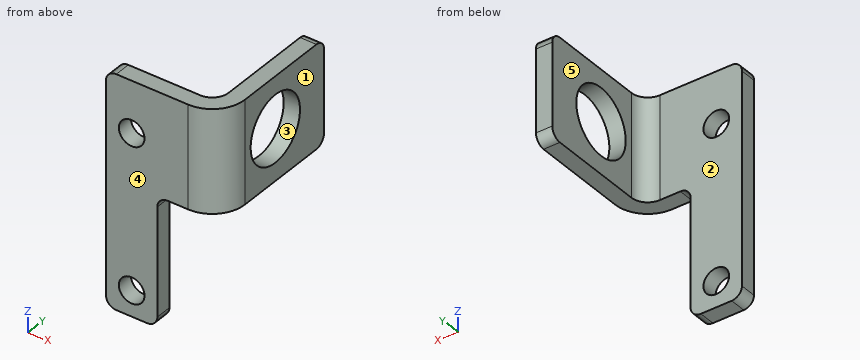
```python
from build123d import *

# Parameters (mm, degrees)
SKETCH2_W           = 10
SKETCH2_H           = 45
BOSS_EXTRUDE1_DEPTH = 3.175
CUT_EXTRUDE1_REACH  = 48.207
SKETCH4_R           = 2.5
EDGE_FLANGE2_DEPTH  = 20
CUT_EXTRUDE2_REACH  = 57.957
SKETCH15_R          = 6.5
FILLET1_R           = 2


# Sheet-metal steps are written as plain solids
with BuildPart() as part:
    # Sketch2 → Boss-Extrude1 (new body)
    with BuildSketch(Plane(origin=(0, 0, 0), x_dir=(1, 0, 0), z_dir=(0, 1, 0))):
        with Locations((5, 22.5)):
            Rectangle(SKETCH2_W, SKETCH2_H)
    extrude(amount=BOSS_EXTRUDE1_DEPTH)

    # Sketch4 → Cut-Extrude1 (cut, up to next)
    with BuildSketch(Plane(origin=(0, 3.175, 0), x_dir=(1, 0, 0), z_dir=(0, 1, 0)), mode=Mode.PRIVATE) as cut_extrude1_sk1:
        with Locations(Location((5, 10, 0), (0, 0, 270))):
            Circle(SKETCH4_R)
    cut_extrude1_tool1 = extrude(cut_extrude1_sk1.sketch, amount=-CUT_EXTRUDE1_REACH, mode=Mode.PRIVATE) & part.part
    # Sketch4 → Cut-Extrude1 (cut, up to next)
    with BuildSketch(Plane(origin=(0, 3.175, 0), x_dir=(1, 0, 0), z_dir=(0, 1, 0)), mode=Mode.PRIVATE) as cut_extrude1_sk2:
        with Locations(Location((5, 40, 0), (0, 0, 270))):
            Circle(SKETCH4_R)
    cut_extrude1_tool2 = extrude(cut_extrude1_sk2.sketch, amount=-CUT_EXTRUDE1_REACH, mode=Mode.PRIVATE) & part.part
    add(cut_extrude1_tool1.solids().sort_by_distance((5, 3.175, -10))[0], mode=Mode.SUBTRACT)
    add(cut_extrude1_tool2.solids().sort_by_distance((5, 3.175, -40))[0], mode=Mode.SUBTRACT)

    # Edge-Flange2 section (across the edge) → Edge-Flange2 (add)
    with BuildSketch(Plane(origin=(19.175, 3.175, 0), x_dir=(-1, 0, 0), z_dir=(0, 0, -1))):
        with BuildLine():
            Line((-3.175, 3.175), (-3.175, 24))
            Line((-3.175, 24), (0, 24))
            Line((0, 24), (0, 3.175))
            ThreePointArc((0, 3.175), (0.92993597, 0.92993597), (3.175, 0))
            Line((3.175, 0), (9.175, 0))
            Line((9.175, 0), (9.175, -3.175))
            Line((9.175, -3.175), (3.175, -3.175))
            ThreePointArc((3.175, -3.175), (-1.315128061, -1.315128061), (-3.175, 3.175))
        make_face()
    extrude(amount=EDGE_FLANGE2_DEPTH)

    # Sketch15 → Cut-Extrude2 (cut, up to next)
    with BuildSketch(Plane.ZY.offset(-19.175), mode=Mode.PRIVATE) as cut_extrude2_sk1:
        with Locations(Location((-10, 14.35, 0), (0, 0, 270))):
            Circle(SKETCH15_R)
    cut_extrude2_tool1 = extrude(cut_extrude2_sk1.sketch, amount=-CUT_EXTRUDE2_REACH, mode=Mode.PRIVATE) & part.part
    add(cut_extrude2_tool1.solids().sort_by_distance((19.175, 14.35, -10))[0], mode=Mode.SUBTRACT)

    # Fillet1
    fillet1_edges = [part.edges().sort_by_distance(p)[0] for p in [
        (0, 1.5875, 0),
        (0, 1.5875, -45),
        (10, 1.5875, -45),
        (10, 1.5875, -20),
        (20.7625, 27.175, 0),
        (20.7625, 27.175, -20),
    ]]
    fillet(fillet1_edges, radius=FILLET1_R)


solid = part.part
```
Part model, mm, in its own coordinate system. Face numbers are marked on the shaded views. A direction names the side the tool comes from. Coordinates: 2 decimals unless noted, no trailing zeros. Order: outer loops, then holes, each group sorted by start corner. A loop starts at its lowest first (then second) coordinate and runs counter-clockwise, first axis right, second up. Notation, with made-up numbers: (42.5, 72) - (76.5, 72) arc R31 cw to (76.5, 111) - close; hole circle Ø11 at (52.5, -39). An arc over 180 degrees is marked (long way). Return JSON: item names as keys, results as strings. Group by question number.
Item 1: Pull direction Y, two halves, no side cores. Call the marked faces 1, 2 and 3: pulls with the +Y half, pulls with the -Y half, needs draft (parallel to the pull), parting line crosses it, or undercut.
Item 2: Pin check, flat tips, straight feed: pin 1 (1.6 mm diameter, centred on y = 1.5, z = -32, fed in from +X); pin 2 (8 mm diameter, centred on x = 5, z = -10, fed in from +Y) (3 decimals). Stop position of each tip, or through.
Item 3: Cut at B-B (z = -40). List the corners of the cut face in (x, y) (3 decimals), plus the area to 3 significant figures.
Item 4: Which spindle directions (+Z, -Z, +X, -X, +Y, -Y) get a long thin tool onto all of the face, cutting with end or side? Do the marked faces 4 and 5. Say none if no direction does.
Item 5: Cut at A-A (x = 5). List the corners of the cut face in (y, z) (3 decimals), plus the area to 3 significant figures.
Item 6: Cut at D-D (z = -10). List the corners of the cut face in (x, y) (3 decimals).
Item 7: Cut at C-C (y = 14.35). List the corners of the cut face in (x, z) (3 decimals).
Item 8: Drill centre lines: probe 1 along X at (y, z) = (1.05, -40); probe 2 along Y at (x, z) = (9, -42) (3 decimals); probe 3 along Y at (x, z) = (21.25, -9) (3 decimals). Where is each one in solid material? Low to high. Write a range as from..to.
Check values:
{
 "1": {"face 1": "needs draft", "face 2": "pulls with the +Y half", "face 3": "undercut"},
 "2": {"pin 1": "stops at x = 10", "pin 2": "stops at y = 3.175"},
 "3": {"outline": "(0, 0) - (2.5, 0) - (2.5, 3.175) - (0, 3.175) - close; (7.5, 0) - (10, 0) - (10, 3.175) - (7.5, 3.175) - close", "area": "15.9 mm2"},
 "4": {"face 4": "+Z, -Z, +X, -X, -Y", "face 5": "+Z, -Z, -X, +Y"},
 "5": {"outline": "(0, -45) - (3.175, -45) - (3.175, -42.5) - (0, -42.5) - close; (0, -37.5) - (3.175, -37.5) - (3.175, -12.5) - (0, -12.5) - close; (0, -7.5) - (3.175, -7.5) - (3.175, 0) - (0, 0) - close", "area": "111 mm2"},
 "6": {"outline": "(0, 0) - (2.5, 0) - (2.5, 3.175) - (0, 3.175) - close; (7.5, 0) - (16, 0) arc R6.35 ccw to (22.35, 6.35) - (22.35, 7.85) - (19.175, 7.85) - (19.175, 6.35) arc R3.175 cw to (16, 3.175) - (7.5, 3.175) - close; (19.175, 20.85) - (22.35, 20.85) - (22.35, 27.175) - (19.175, 27.175) - close"},
 "7": {"outline": "(19.175, -20) - (22.35, -20) - (22.35, -16.5) - (19.175, -16.5) - close; (19.175, -3.5) - (22.35, -3.5) - (22.35, 0) - (19.175, 0) - close"},
 "8": {"probe 1": "x = 0..2.5, 7.5..10", "probe 2": "y = 0..3.175", "probe 3": "y = 2.778..7.927, 20.773..27.175"}
}
